from build123d import *

# Parameters (mm, degrees)
SKETCH1_R           = 200
BOSS_EXTRUDE1_DEPTH = 8
SKETCH2_R           = 190
BOSS_EXTRUDE2_DEPTH = 175
SKETCH3_R           = 225
BOSS_EXTRUDE3_DEPTH = 8
SKETCH4_R           = 187
CUT_EXTRUDE1_DEPTH  = 175
SKETCH5_R           = 200
SKETCH5_R_2         = 192.2
CUT_EXTRUDE2_DEPTH  = 4.6
SKETCH6_R           = 5.25
CUT_EXTRUDE3_DEPTH  = 10
CIRPATTERN1_COUNT   = 17


with BuildPart() as part:
    # Sketch1 → Boss-Extrude1 (new body)
    with BuildSketch(Plane(origin=(0, 0, 0), x_dir=(1, 0, 0), z_dir=(0, 1, 0))):
        with Locations(Location((0, 0, 0), (0, 0, 270))):
            Circle(SKETCH1_R)
    extrude(amount=-BOSS_EXTRUDE1_DEPTH)

    # Sketch2 → Boss-Extrude2 (add)
    with BuildSketch(Plane(origin=(0, 0, 0), x_dir=(1, 0, 0), z_dir=(0, 1, 0))):
        with Locations(Location((0, 0, 0), (0, 0, 270))):
            Circle(SKETCH2_R)
    extrude(amount=BOSS_EXTRUDE2_DEPTH)

    # Sketch3 → Boss-Extrude3 (add)
    with BuildSketch(Plane(origin=(0, 175, 0), x_dir=(1, 0, 0), z_dir=(0, 1, 0))):
        with Locations(Location((0, 0, 0), (0, 0, 270))):
            Circle(SKETCH3_R)
    extrude(amount=-BOSS_EXTRUDE3_DEPTH)

    # Sketch4 → Cut-Extrude1 (cut)
    with BuildSketch(Plane(origin=(0, 175, 0), x_dir=(1, 0, 0), z_dir=(0, 1, 0))):
        with Locations(Location((0, 0, 0), (0, 0, 270))):
            Circle(SKETCH4_R)
    extrude(amount=-CUT_EXTRUDE1_DEPTH, mode=Mode.SUBTRACT)

    # Sketch5 → Cut-Extrude2 (cut)
    with BuildSketch(Plane(origin=(0, 175, 0), x_dir=(1, 0, 0), z_dir=(0, 1, 0))):
        with Locations(Location((0, 0, 0), (0, 0, 270))):
            Circle(SKETCH5_R)
        with Locations(Location((0, 0, 0), (0, 0, 270))):
            Circle(SKETCH5_R_2, mode=Mode.SUBTRACT)
    extrude(amount=-CUT_EXTRUDE2_DEPTH, mode=Mode.SUBTRACT)

    # Sketch6 → Cut-Extrude3 (cut)
    with BuildSketch(Plane(origin=(0, 175, 0), x_dir=(1, 0, 0), z_dir=(0, 1, 0))):
        with Locations(Location((0, 210, 0), (0, 0, 270))):
            Circle(SKETCH6_R)
    cut_extrude3 = extrude(amount=-CUT_EXTRUDE3_DEPTH, mode=Mode.SUBTRACT)

    # CirPattern1: Cut-Extrude3 ×17 about axis
    cirpattern1_axis = Axis((0, 0, 0), (0, 1, 0))
    for i in range(1, CIRPATTERN1_COUNT):
        add(cut_extrude3.rotate(cirpattern1_axis, i * 360 / CIRPATTERN1_COUNT), mode=Mode.SUBTRACT)


solid = part.part
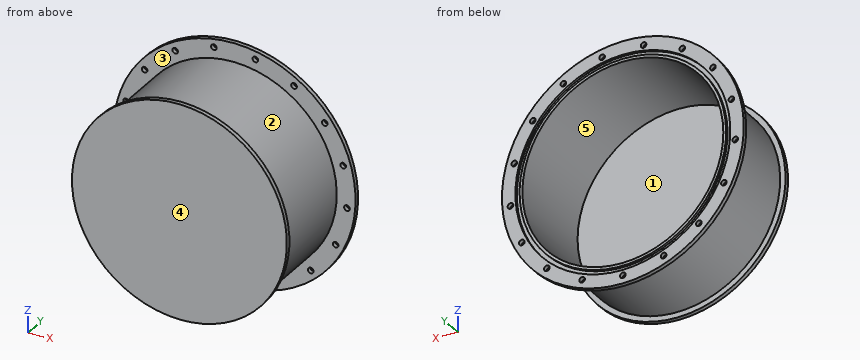
Geometry check sheet. Reference: the model listing, model coordinates, mm. Face numbers are marked on the shaded views. A direction names the side the tool comes from. Coordinates: 2 decimals unless noted, no trailing zeros. Order: outer loops, then holes, each group sorted by start corner. A loop starts at its lowest first (then second) coordinate and runs counter-clockwise, first axis right, second up. Notation, with made-up numbers: (-7, 64.25) -> (21, 64.25) arc R15 ccw to (21, 78.25) -> close; hole circle Ø9 at (15, 42). An arc over 180 degrees is marked (long way). Use a Markdown table: item, result. Add a question column.
1. Cross-section at C-C (x = 90). Enter the section's corners in (y, z), and give its area (3 significant figures).
2. Set-up check for the marked faces 4 and 5: record each of +Z, -Z, +X, -X, +Y, -Y from which the full face is reachable in a straight line by a thin tool's end or side.
3. Cross-section at B-B (y = 99). Enter the section's corners in (x, z), and give its area (3 significant figures).
4. Material ranges on L1, parallel to Y at x = 35, z = 195; L2, parallel to Y at x = 179, z = 66; L3, parallel to Y at x = -55, z = -54.5, recorded low to high.
5. Go/stop test with flat-tipped pins: pin 1 Ø13.5 at (x, z) = (-167.58, 126.55) entering from -Y; pin 2 Ø6 at (x, z) = (-136.5, -107.5) entering from +Y; pin 3 Ø8.5 at (x, z) = (38.59, 206.42) entering from -Y; pin 4 Ø6 at (y, z) = (22, 106) entering from +X. Record where each tip stops, or that it passes through.
6. Mould release check, pull along Z, two halves, no side actions. Record for the marked faces 1, 2 and 3: pulls with the +Z half, pulls with the -Z half, needs draft (parallel to the pull), parting line crosses it, or undercut.
7. Cross-section at A-A (z = 0). Enter the section's corners in (x, y).
Filled sheet:
| question | item | result |
|---|---|---|
| 1 | outline | (-8, -178.61) -> (0, -178.61) -> (0, -167.33) -> (167, -167.33) -> (167, -206.22) -> (175, -206.22) -> (175, -178.61) -> (170.4, -178.61) -> (170.4, -169.83) -> (175, -169.83) -> (175, -163.92) -> (0, -163.92) -> (0, 163.92) -> (175, 163.92) -> (175, 169.83) -> (170.4, 169.83) -> (170.4, 178.61) -> (175, 178.61) -> (175, 206.22) -> (167, 206.22) -> (167, 167.33) -> (0, 167.33) -> (0, 178.61) -> (-8, 178.61) -> close |
| 1 | area | 4,590 mm2 |
| 2 | face 4 | +Z, -Z, +X, -X, -Y |
| 2 | face 5 | +Y |
| 3 | outline | circle Ø380 at (0, 0); hole circle Ø374 at (0, 0) |
| 3 | area | 3,550 mm2 |
| 4 | L1 | -8 to 0, 167 to 170.4 |
| 4 | L2 | -8 to 0, 167 to 175 |
| 4 | L3 | -8 to 0 |
| 5 | pin 1 | y = 167 |
| 5 | pin 2 | y = 0 |
| 5 | pin 3 | through |
| 5 | pin 4 | x = 159.66 |
| 6 | face 1 | undercut |
| 6 | face 2 | parting line crosses it |
| 6 | face 3 | needs draft |
| 7 | outline | (-225, 167) -> (-190, 167) -> (-190, 0) -> (-200, 0) -> (-200, -8) -> (200, -8) -> (200, 0) -> (190, 0) -> (190, 167) -> (225, 167) -> (225, 175) -> (200, 175) -> (200, 170.4) -> (192.2, 170.4) -> (192.2, 175) -> (187, 175) -> (187, 0) -> (-187, 0) -> (-187, 175) -> (-192.2, 175) -> (-192.2, 170.4) -> (-200, 170.4) -> (-200, 175) -> (-225, 175) -> close |
